Part model, mm, in its own coordinate system. Face numbers are marked on the shaded views. Give positions to 0.01 mm unless a question says otherwise; leave off trailing zeros. Order: outer loops, then holes, each group sorted by start corner. A loop starts at its lowest first (then second) coordinate and runs counter-clockwise, first axis right, second up. Notation, with made-up numbers: (33.25, -32) -> (46.25, -32) arc R28 cw to (46.25, 6) -> close; hole circle Ø6 at (35, 58). An arc over 180 degrees is marked (long way). Write item = value, one per line. Start each with the question number.
(1) Probe line 1 along Y through (x, z) = (155, 39.75) (3 decimals); line 2 along Y through (x, z) = (157, 41); line 3 along X through (y, z) = (-25, 42.25) (3 decimals). List the from-to ranges inside material, lowest first. Write a range as from..to.
(2) Saw through at A-A, the plane y = -25. List the corners of the cut face in (x, z) (3 decimals).
(3) Two-plate mould, pull along Y, no slides. Class the marked faces 1, 2 and 3: pulls with the +Y half, pulls with the -Y half, needs draft (parallel to the pull), parting line crosses it, or undercut.
(4) Saw through at C-C, the plane z = 45. List the corners of the cut face in (x, y) (3 decimals), then the cut area to 3 significant figures.
(5) Saw through at D-D, the plane x = 165.5. List the corners of the cut face in (y, z), then the cut area to 3 significant figures.
(6) Flat gauge pins, fed straight in: pin 1 (8 mm diameter, centred on x = 155, y = -25, fed in from -Z); pin 2 (4 mm diameter, centred on x = 155, y = -7, fed in from +Z). Where does each tip first touch, or does it go through?
(7) Saw through at B-B, the plane x = 155. List the corners of the cut face in (y, z) (3 decimals).
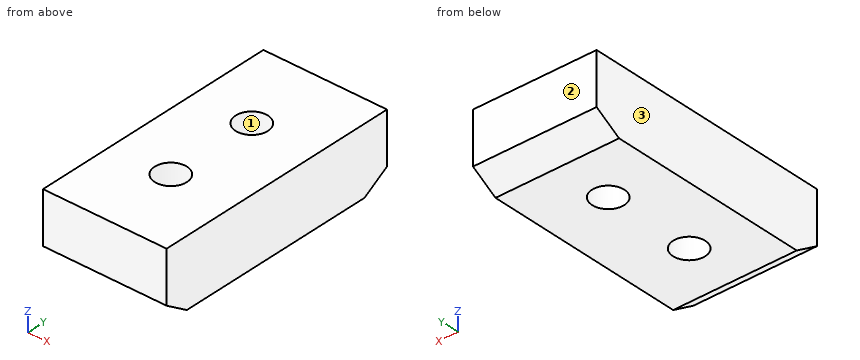
from build123d import *

# Parameters (mm, degrees)
PAD001_DEPTH    = 24
SKETCH021_R     = 3.125
POCKET019_DEPTH = 49.001


with BuildPart() as part:
    # Sketch020 → Pad001 (new body)
    with BuildSketch(Plane.YZ.offset(143.5)):
        Polygon((-40.25, 49), (8.75, 49), (8.75, 39), (3.75, 36), (-35.75, 36), (-40.25, 39), align=None)
    extrude(amount=PAD001_DEPTH)

    # Sketch021 → Pocket019 (cut, through all)
    with BuildSketch(Plane.XY):
        with Locations((155, -7)):
            Circle(SKETCH021_R)
        with Locations((155, -25)):
            Circle(SKETCH021_R)
    extrude(amount=POCKET019_DEPTH, mode=Mode.SUBTRACT)


solid = part.part
Results list:
q1.line_1 = -40.25..-28.125, -21.875..-10.125, -3.875..8.75
q1.line_2 = -40.25..-27.4, -22.6..-9.4, -4.6..8.75
q1.line_3 = 143.5..151.875, 158.125..167.5
q2.outline = (143.5, 36) -> (151.875, 36) -> (151.875, 49) -> (143.5, 49) -> close; (158.125, 36) -> (167.5, 36) -> (167.5, 49) -> (158.125, 49) -> close
q3.face_1 = undercut
q3.face_2 = pulls with the +Y half
q3.face_3 = needs draft
q4.outline = (143.5, -40.25) -> (167.5, -40.25) -> (167.5, 8.75) -> (143.5, 8.75) -> close; hole circle Ø6.25 at (155, -25); hole circle Ø6.25 at (155, -7)
q4.area = 1,110 mm^2
q5.outline = (-40.25, 39) -> (-35.75, 36) -> (3.75, 36) -> (8.75, 39) -> (8.75, 49) -> (-40.25, 49) -> close
q5.area = 623 mm^2
q6.pin_1 = 36
q6.pin_2 = through
q7.outline = (-40.25, 39) -> (-35.75, 36) -> (-28.125, 36) -> (-28.125, 49) -> (-40.25, 49) -> close; (-21.875, 36) -> (-10.125, 36) -> (-10.125, 49) -> (-21.875, 49) -> close; (-3.875, 36) -> (3.75, 36) -> (8.75, 39) -> (8.75, 49) -> (-3.875, 49) -> close
